from build123d import *

# Parameters (mm, degrees)
F2_DEPTH = 8


with BuildPart() as f2:
    # F1 (on Top) → F2 (new body)
    with BuildSketch(Plane.XY):
        with BuildLine():
            ThreePointArc((4.954369, 6.121262), (7.672943, 1.772448), (7.137174, -3.328119))
            ThreePointArc((7.137174, -3.328119), (8.104553, -5.985971), (10.762405, -5.018592))
            ThreePointArc((10.762405, -5.018592), (11.706561, 1.993), (8.495444, 8.297172))
            ThreePointArc((8.495444, 8.297172), (7.508107, 9.749502), (7.083848, 11.453644))
            ThreePointArc((7.083848, 11.453644), (0, 18.075), (-7.083848, 11.453644))
            ThreePointArc((-7.083848, 11.453644), (-7.508107, 9.749502), (-8.495444, 8.297172))
            ThreePointArc((-8.495444, 8.297172), (-11.706561, 1.993), (-10.762405, -5.018592))
            ThreePointArc((-10.762405, -5.018592), (-8.104553, -5.985971), (-7.137174, -3.328119))
            ThreePointArc((-7.137174, -3.328119), (-7.672943, 1.772448), (-4.954369, 6.121262))
            ThreePointArc((-4.954369, 6.121262), (-3.587343, 7.854659), (-3.1, 10.007778))
            Line((-3.1, 10.007778), (-3.1, 10.975))
            ThreePointArc((-3.1, 10.975), (0, 14.075), (3.1, 10.975))
            Line((3.1, 10.975), (3.1, 10.007778))
            ThreePointArc((3.1, 10.007778), (3.587343, 7.854659), (4.954369, 6.121262))
        make_face()
    extrude(amount=F2_DEPTH)


solid = f2.part
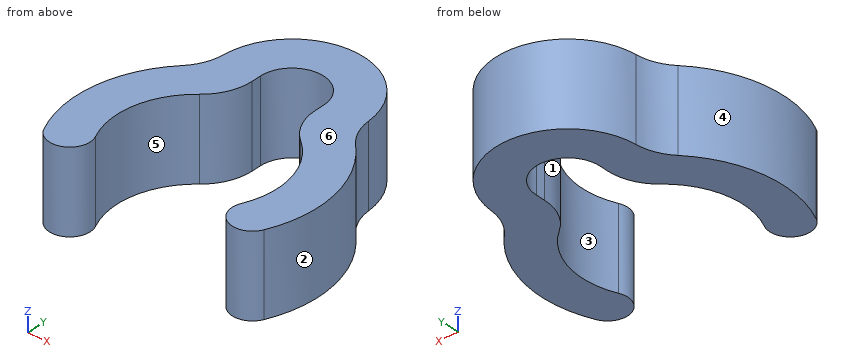
Work out the finished part from the listing and answer in its coordinate system (mm). Face numbers are marked on the shaded views. A direction names the side the tool comes from. Round coordinates to 2 decimals unless told otherwise and drop trailing zeros. Loops run counter-clockwise (first coordinate to the right, second up) from the corner with the lowest first, then second, coordinate; pieces in that order, holes last. Notation, with made-up numbers: M 60.5,78.5 L 75.5,78.5 A38 cw 75.5,117.5 Z; hole C -12.75,12.5 d4. An arc over 180 degrees is marked long. One line per question, with ' | ' between items. Start each with the question number.
(1) Flat-ended cylindrical pins translate along their axes: pin 1 Ø0.8 at (y, z) = (10.5, 3) entering from +X; pin 2 Ø0.8 at (y, z) = (10.5, 5) entering from -X; pin 3 Ø1.5 at (y, z) = (2, 4) entering from -X. Find the tip coordinate at first contact, or state that the pin passes through.
(2) A tool of negligible diameter and unlimited length cuts with its end or side. For the marked faces 1, 2 and 3, from which of +Z, -Z, +X, -X, +Y, -Y can it reach the whole face along a straight path? Write none if from no direction.
(3) A cutting plane is placed at C-C on y = 14.5. Write down the section's boundary in (x, z), plus the area to 3 significant figures.
(4) A cutting plane is placed at A-A on x = 0. Write down the section's boundary in (y, z) (3 decimals).
(5) Find the intervals of material crossed by line 1 (X direction, y = 4.5, z = 0.5); line 2 (X direction, y = 1.75, z = 5); line 3 (X direction, y = 15.25, z = 0.5), in increasing order.
(6) A cutting plane is placed at B-B on z = 3. Write down the section's boundary in (x, y) (3 decimals).
(7) For a pull along X with two mould halves and no side action, classify the marked faces 4, 5 and 6 as released by +X, released by -X, zero draft, split by the parting line, or undercut.
Geometry check:
1) pin 1: stops at x = 7.37 | pin 2: stops at x = -7.37 | pin 3: stops at x = -11.81
2) face 1: +Z, -Z, -Y | face 2: +Z, -Z, +X | face 3: +Z, -Z
3) outline: M -6.16,0 L 6.16,0 L 6.16,8 L -6.16,8 Z | area: 98.6 mm²
4) outline: M 14.075,0 L 18.075,0 L 18.075,8 L 14.075,8 Z
5) line 1: x = -10.99 to -6.46, 6.46 to 10.99 | line 2: x = -11.75 to -7.68, 7.68 to 11.75 | line 3: x = -5.67 to 5.67
6) outline: M -10.762,-5.019 A2 ccw -7.137,-3.328 A7.875 cw -4.954,6.121 A5 ccw -3.1,10.008 L -3.1,10.975 A3.1 cw 3.1,10.975 L 3.1,10.008 A5 ccw 4.954,6.121 A7.875 cw 7.137,-3.328 A2 ccw 10.762,-5.019 A11.875 ccw 8.495,8.297 A5 cw 7.084,11.454 A7.1 ccw -7.084,11.454 A5 cw -8.495,8.297 A11.875 ccw Z
7) face 4: released by -X | face 5: undercut | face 6: zero draft
